from build123d import *

# Parameters (mm, degrees)
ESBO_O1_R                = 2.79
RESSALTO_EXTRUS_O1_DEPTH = 161


with BuildPart() as part:
    # Esboço1 → Ressalto-extrusão1 (new body)
    with BuildSketch(Plane(origin=(0, 85, 0), x_dir=(1, 0, 0), z_dir=(0, 1, 0))):
        with BuildLine():
            Line((6.162658774, -1.825961894), (7.216878365, 0))
            Line((7.216878365, 0), (6.162658774, 1.825961894))
            ThreePointArc((6.162658774, 1.825961894), (4.113620668, 2.375), (4.662658774, 4.424038106))
            Line((4.662658774, 4.424038106), (3.608439182, 6.25))
            Line((3.608439182, 6.25), (1.5, 6.25))
            ThreePointArc((1.5, 6.25), (0, 4.75), (-1.5, 6.25))
            Line((-1.5, 6.25), (-3.608439182, 6.25))
            Line((-3.608439182, 6.25), (-4.662658774, 4.424038106))
            ThreePointArc((-4.662658774, 4.424038106), (-4.113620668, 2.375), (-6.162658774, 1.825961894))
            Line((-6.162658774, 1.825961894), (-7.216878365, 0))
            Line((-7.216878365, 0), (-6.162658774, -1.825961894))
            ThreePointArc((-6.162658774, -1.825961894), (-4.113620668, -2.375), (-4.662658774, -4.424038106))
            Line((-4.662658774, -4.424038106), (-3.608439182, -6.25))
            Line((-3.608439182, -6.25), (-1.5, -6.25))
            ThreePointArc((-1.5, -6.25), (0, -4.75), (1.5, -6.25))
            Line((1.5, -6.25), (3.608439182, -6.25))
            Line((3.608439182, -6.25), (4.662658774, -4.424038106))
            ThreePointArc((4.662658774, -4.424038106), (4.113620668, -2.375), (6.162658774, -1.825961894))
        make_face()
        Circle(ESBO_O1_R, mode=Mode.SUBTRACT)
    extrude(amount=-RESSALTO_EXTRUS_O1_DEPTH)


solid = part.part
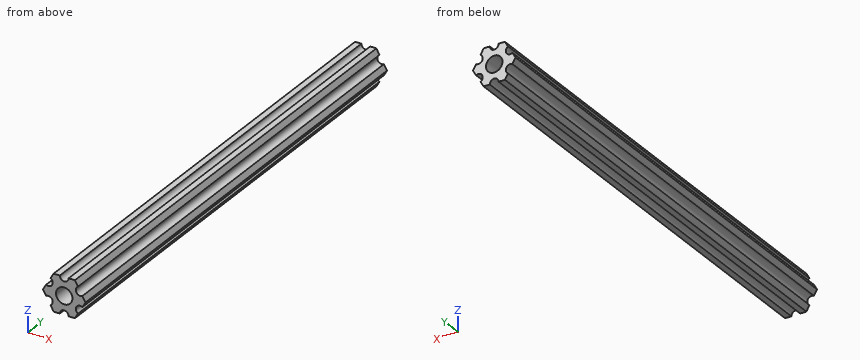
The model under review builds one solid part; all positions refer to its coordinate system, in mm. Coordinates: 2 decimals unless noted, no trailing zeros. Write each loop counter-clockwise with the first axis right and the second up, starting at its lowest first coordinate (ties: lowest second). Pieces come first, ordered by that corner, then holes. Notation, with made-up numbers: (57, -3.5) - (66, -3.5) arc R21 ccw to (66, 3.5) - close; hole circle Ø4 at (77.5, 10.25). An arc over 180 degrees is marked (long way). Answer as a JSON object with one key per item and string values. Group by question number.
1. Add section A-A (x = 0). Give the boundary of the cut face in (y, z), plus the area to 3 significant figures.
2. To check wall thickness, follow probe 1 along Z at (x, y) = (0, 42.5); probe 2 along X at (y, z) = (-63.5, 0.5); probe 3 along X at (y, z) = (-25.5, -5). State the ranges of each line that lie inside material, in increasing order.
3. Clearance check with flat-ended pins moving along their axes: pin 1 Ø5 at (y, z) = (65.5, -4) entering from -X; pin 2 Ø8 at (x, y) = (-4.5, -34.5) entering from -Z. State where each tip first meets the part, or that it passes through.
Findings:
{
 "1": {"outline": "(-76, -4.75) - (85, -4.75) - (85, -2.79) - (-76, -2.79) - close; (-76, 2.79) - (85, 2.79) - (85, 4.75) - (-76, 4.75) - close", "area": "631 mm²"},
 "2": {"probe 1": "-4.75 to -2.79, 2.79 to 4.75", "probe 2": "-6.93 to -2.74, 2.74 to 6.93", "probe 3": "-4.33 to -0.83, 0.83 to 4.33"},
 "3": {"pin 1": "x = -6.35", "pin 2": "z = -6.25"}
}
